Autodesk Fusion 360 part; units mm, degrees
sketch "Sketch1" plane through (0, 0, 0) normal (0, 0, 1) x (1, 0, 0)
  circle A0 centre (0, 0) radius 9.5
  circle A1 centre (0, 0) radius 7.5
  line L0 (4.1569, 0) -> (2.0785, 3.6)
  line L1 (2.0785, 3.6) -> (-2.0785, 3.6)
  line L2 (-2.0785, 3.6) -> (-4.1569, 0)
  line L3 (-4.1569, 0) -> (-2.0785, -3.6)
  line L4 (-2.0785, -3.6) -> (2.0785, -3.6)
  line L5 (2.0785, -3.6) -> (4.1569, 0)
  line L6 (-4.1569, 0) -> (4.1569, 0) construction
  dimension "d1" = 19
  dimension "d2" = 15
  dimension "d3" = 7.2
extrude "Extrude1" add sketch "Sketch1" along normal blind 0.5 contours A1
extrude "Extrude2" [suppressed]
extrude "Extrude3" [suppressed]
Verification items for the finished model (mm, model axes). A direction names the side the tool comes from. Give positions to 0.01 mm unless a question says otherwise; leave off trailing zeros. Order: outer loops, then holes, each group sorted by start corner. A loop starts at its lowest first (then second) coordinate and runs counter-clockwise, first axis right, second up. Notation, with made-up numbers: (-30.5, 76.5) -> (-22.5, 76.5) arc R29 cw to (-22.5, 100.5) -> close; hole circle Ø9 at (37, 57). An arc over 180 degrees is marked (long way). One line per item, written item: value.
(1) Gauge pin test, flat end, axial feed: pin 1 (3 mm diameter, centred on x = -2, y = 0, fed in from +Z). Record the tip position at first contact, or that the pin passes through.
Final values:
pin 1: through
(2) Scan lines: line 1 along Y through (x, z) = (0, 0.45); line 2 along X through (y, z) = (0.25, 0.3); line 3 along X through (y, z) = (2.75, 0.05). Record each from-to range of solid material in increasing order. Write a range as [from, to].
Final values:
line 1: [-7.5, -3.6], [3.6, 7.5]
line 2: [-7.5, -4.01], [4.01, 7.5]
line 3: [-6.98, -2.57], [2.57, 6.98]
(3) Sectioned sample at D-D on x = 5.25. Record the cut outline in (y, z).
Final values:
outline: (-5.36, 0) -> (5.36, 0) -> (5.36, 0.5) -> (-5.36, 0.5) -> close
(4) Sectioned sample at C-C on y = -1.25. Record the cut outline in (x, z), then the cut area to 3 significant figures.
Final values:
outline: (-7.4, 0) -> (-3.44, 0) -> (-3.44, 0.5) -> (-7.4, 0.5) -> close; (3.44, 0) -> (7.4, 0) -> (7.4, 0.5) -> (3.44, 0.5) -> close
area: 3.96 mm^2
(5) Tool access check on faces 1 (the face through (-3.44, -1.56, 0)), 2 (the face through (3.1, -1.83, 0.25)). Record the directions out of +Z, -Z, +X, -X, +Y, -Y that give a thin tool (end or side, any length) a straight path to the whole face; none if there is none.
Final values:
face 1: -Z, +X, -X, +Y, -Y
face 2: +Z, -Z
(6) Draft check along Y on faces 3 (the face through (-7.493, -0.33, 0.246)), 4 (the face through (3.132, 1.775, 0.246)), 5 (the face through (-3.44, -1.56, 0.5)). Enter one of: pulls with the +Y half, pulls with the -Y half, needs draft (parallel to the pull), parting line crosses it, or undercut.
Final values:
face 3: parting line crosses it
face 4: undercut
face 5: needs draft
(7) Sectioned sample at A-A on x = 0. Record the cut outline in (y, z), then the cut area to 3 significant figures.
Final values:
outline: (-7.5, 0) -> (-3.6, 0) -> (-3.6, 0.5) -> (-7.5, 0.5) -> close; (3.6, 0) -> (7.5, 0) -> (7.5, 0.5) -> (3.6, 0.5) -> close
area: 3.90 mm^2
(8) Sectioned sample at B-B on z = 0.2. Record the cut outline in (x, y), then the cut area to 3 significant figures.
Final values:
outline: circle Ø15 at (0, 0); hole (-4.16, 0) -> (-2.08, -3.6) -> (2.08, -3.6) -> (4.16, 0) -> (2.08, 3.6) -> (-2.08, 3.6) -> close
area: 132 mm^2
